from build123d import *

# Parameters (mm, degrees)
SKETCH1_R                       = 7.7978
SKETCH1_R_2                     = 6.57225
SKETCH1_R_3                     = 5.17525
BOSS_EXTRUDE1_DEPTH             = 2.032
BOSS_EXTRUDE2_REACH             = 17.062
BOSS_EXTRUDE2_DIRECTION_2_REACH = 17.062
SKETCH4_W                       = 3.302
SKETCH4_H                       = 2.032
BOSS_EXTRUDE3_DEPTH             = 30.1244
FILLET1_R                       = 2.54
FILLET2_R                       = 2.54
SKETCH5_W                       = 9.0678
SKETCH5_H                       = 2.54
CUT_EXTRUDE1_DEPTH              = 116.84
SKETCH6_R                       = 2.01295
CUT_EXTRUDE2_DEPTH              = 5.7117
SKETCH7_R                       = 1.524
CUT_EXTRUDE3_DEPTH              = 26.9207
CUT_EXTRUDE4_DEPTH              = 116.84
CUT_EXTRUDE4_DEPTH_BACK         = 116.84
SKETCH9_W                       = 42.5577
SKETCH9_H                       = 30.1244
SKETCH9_W_2                     = 39.0017
SKETCH9_H_2                     = 26.5684
BOSS_EXTRUDE4_DEPTH             = 1.778


with BuildPart() as part:
    # Sketch1 → Boss-Extrude1 (new body)
    with BuildSketch(Plane(origin=(0, 0, 0), x_dir=(1, 0, 0), z_dir=(0, 1, 0))):
        with BuildLine():
            ThreePointArc((-23.05685, 9.9822), (-21.568952448, 13.574302448), (-17.97685, 15.0622))
            Line((-17.97685, 15.0622), (17.97685, 15.0622))
            ThreePointArc((17.97685, 15.0622), (21.568952448, 13.574302448), (23.05685, 9.9822))
            Line((23.05685, 9.9822), (23.05685, -9.9822))
            ThreePointArc((23.05685, -9.9822), (21.568952448, -13.574302448), (17.97685, -15.0622))
            Line((17.97685, -15.0622), (-17.97685, -15.0622))
            ThreePointArc((-17.97685, -15.0622), (-21.568952448, -13.574302448), (-23.05685, -9.9822))
            Line((-23.05685, -9.9822), (-23.05685, 9.9822))
        make_face()
        Circle(SKETCH1_R, mode=Mode.SUBTRACT)
        Circle(SKETCH1_R)
        Circle(SKETCH1_R_2, mode=Mode.SUBTRACT)
        Circle(SKETCH1_R_2)
        Circle(SKETCH1_R_3, mode=Mode.SUBTRACT)
    extrude(amount=-BOSS_EXTRUDE1_DEPTH)

    # Sketch2 → Revolve1 (revolve)
    with BuildSketch(Plane(origin=(0, 0, 0), x_dir=(0, 0, -1), z_dir=(1, 0, 0))):
        Polygon((-5.17525, 2.286), (-6.57225, 2.794), (-7.7978, 0), (-5.17525, 0), align=None)
    revolve1 = revolve(axis=Axis((0, 0, 0), (0, 1, 0)))

    # Boss-Extrude2: up to this face of the body (flat: up to its plane)
    boss_extrude2_end = Plane(part.part.faces().sort_by_distance((0, -1.016, 15.0622))[0])
    # Sketch3 → Boss-Extrude2 (add, up to the picked face)
    with BuildSketch(Plane.XY, mode=Mode.PRIVATE) as boss_extrude2_sk1:
        with BuildLine():
            ThreePointArc((-23.05685, -1.27), (-22.684875612, -0.371974388), (-21.78685, 0))
            Line((-21.78685, 0), (-21.27885, 0))
            Line((-21.27885, 0), (-21.27885, -21.717))
            ThreePointArc((-21.27885, -21.717), (-21.650824388, -22.615025612), (-22.54885, -22.987))
            Line((-22.54885, -22.987), (-23.05685, -22.987))
            Line((-23.05685, -22.987), (-32.16275, -22.987))
            Line((-32.16275, -22.987), (-32.16275, -25.9207))
            Line((-32.16275, -25.9207), (-33.94075, -25.9207))
            Line((-33.94075, -25.9207), (-33.94075, -22.479))
            ThreePointArc((-33.94075, -22.479), (-33.568775612, -21.580974388), (-32.67075, -21.209))
            Line((-32.67075, -21.209), (-32.16275, -21.209))
            Line((-32.16275, -21.209), (-23.05685, -21.209))
            Line((-23.05685, -21.209), (-23.05685, -1.27))
        make_face()
    boss_extrude2_tool1 = split(extrude(boss_extrude2_sk1.sketch, amount=BOSS_EXTRUDE2_REACH, mode=Mode.PRIVATE), bisect_by=boss_extrude2_end, keep=Keep.BOTH, mode=Mode.PRIVATE)
    add(boss_extrude2_tool1.solids().sort_by_distance((-32.41675, -21.49748, 0))[0])
    # Sketch3 → Boss-Extrude2 (add, up to the picked face)
    with BuildSketch(Plane.XY, mode=Mode.PRIVATE) as boss_extrude2_sk2:
        with BuildLine():
            Line((21.27885, 0), (21.27885, -21.717))
            ThreePointArc((21.27885, -21.717), (21.650824388, -22.615025612), (22.54885, -22.987))
            Line((22.54885, -22.987), (23.05685, -22.987))
            Line((23.05685, -22.987), (32.16275, -22.987))
            Line((32.16275, -22.987), (32.16275, -25.9207))
            Line((32.16275, -25.9207), (33.94075, -25.9207))
            Line((33.94075, -25.9207), (33.94075, -22.479))
            ThreePointArc((33.94075, -22.479), (33.568775612, -21.580974388), (32.67075, -21.209))
            Line((32.67075, -21.209), (32.16275, -21.209))
            Line((32.16275, -21.209), (23.05685, -21.209))
            Line((23.05685, -21.209), (23.05685, -1.27))
            ThreePointArc((23.05685, -1.27), (22.684875612, -0.371974388), (21.78685, 0))
            Line((21.78685, 0), (21.27885, 0))
        make_face()
    boss_extrude2_tool2 = split(extrude(boss_extrude2_sk2.sketch, amount=BOSS_EXTRUDE2_REACH, mode=Mode.PRIVATE), bisect_by=boss_extrude2_end, keep=Keep.BOTH, mode=Mode.PRIVATE)
    add(boss_extrude2_tool2.solids().sort_by_distance((32.41675, -21.49748, 0))[0])

    # Boss-Extrude2 direction 2: up to this face of the body (flat: up to its plane)
    boss_extrude2_direction_2_end = Plane(part.part.faces().sort_by_distance((0, -1.016, -15.0622))[0])
    # Sketch3 → Boss-Extrude2 direction 2 (add, up to the picked face)
    with BuildSketch(Plane.XY, mode=Mode.PRIVATE) as boss_extrude2_direction_2_sk1:
        with BuildLine():
            ThreePointArc((-23.05685, -1.27), (-22.684875612, -0.371974388), (-21.78685, 0))
            Line((-21.78685, 0), (-21.27885, 0))
            Line((-21.27885, 0), (-21.27885, -21.717))
            ThreePointArc((-21.27885, -21.717), (-21.650824388, -22.615025612), (-22.54885, -22.987))
            Line((-22.54885, -22.987), (-23.05685, -22.987))
            Line((-23.05685, -22.987), (-32.16275, -22.987))
            Line((-32.16275, -22.987), (-32.16275, -25.9207))
            Line((-32.16275, -25.9207), (-33.94075, -25.9207))
            Line((-33.94075, -25.9207), (-33.94075, -22.479))
            ThreePointArc((-33.94075, -22.479), (-33.568775612, -21.580974388), (-32.67075, -21.209))
            Line((-32.67075, -21.209), (-32.16275, -21.209))
            Line((-32.16275, -21.209), (-23.05685, -21.209))
            Line((-23.05685, -21.209), (-23.05685, -1.27))
        make_face()
    boss_extrude2_direction_2_tool1 = split(extrude(boss_extrude2_direction_2_sk1.sketch, amount=-BOSS_EXTRUDE2_DIRECTION_2_REACH, mode=Mode.PRIVATE), bisect_by=boss_extrude2_direction_2_end, keep=Keep.BOTH, mode=Mode.PRIVATE)
    add(boss_extrude2_direction_2_tool1.solids().sort_by_distance((-32.41675, -21.49748, 0))[0])
    # Sketch3 → Boss-Extrude2 direction 2 (add, up to the picked face)
    with BuildSketch(Plane.XY, mode=Mode.PRIVATE) as boss_extrude2_direction_2_sk2:
        with BuildLine():
            Line((21.27885, 0), (21.27885, -21.717))
            ThreePointArc((21.27885, -21.717), (21.650824388, -22.615025612), (22.54885, -22.987))
            Line((22.54885, -22.987), (23.05685, -22.987))
            Line((23.05685, -22.987), (32.16275, -22.987))
            Line((32.16275, -22.987), (32.16275, -25.9207))
            Line((32.16275, -25.9207), (33.94075, -25.9207))
            Line((33.94075, -25.9207), (33.94075, -22.479))
            ThreePointArc((33.94075, -22.479), (33.568775612, -21.580974388), (32.67075, -21.209))
            Line((32.67075, -21.209), (32.16275, -21.209))
            Line((32.16275, -21.209), (23.05685, -21.209))
            Line((23.05685, -21.209), (23.05685, -1.27))
            ThreePointArc((23.05685, -1.27), (22.684875612, -0.371974388), (21.78685, 0))
            Line((21.78685, 0), (21.27885, 0))
        make_face()
    boss_extrude2_direction_2_tool2 = split(extrude(boss_extrude2_direction_2_sk2.sketch, amount=-BOSS_EXTRUDE2_DIRECTION_2_REACH, mode=Mode.PRIVATE), bisect_by=boss_extrude2_direction_2_end, keep=Keep.BOTH, mode=Mode.PRIVATE)
    add(boss_extrude2_direction_2_tool2.solids().sort_by_distance((32.41675, -21.49748, 0))[0])

    # Sketch4 → Boss-Extrude3 (add)
    with BuildSketch(Plane.XY.offset(15.0622)):
        with BuildLine():
            ThreePointArc((-23.05685, -1.27), (-22.684875612, -0.371974388), (-21.78685, 0))
            Line((-21.78685, 0), (-23.05685, 0))
            Line((-23.05685, 0), (-23.05685, -1.27))
        make_face()
        with BuildLine():
            Line((-21.27885, -2.032), (-21.27885, 0))
            Line((-21.27885, 0), (-21.78685, 0))
            ThreePointArc((-21.78685, 0), (-22.684875612, -0.371974388), (-23.05685, -1.27))
            Line((-23.05685, -1.27), (-23.05685, -2.032))
            Line((-23.05685, -2.032), (-21.27885, -2.032))
        make_face()
        with Locations((-19.62785, -1.016)):
            Rectangle(SKETCH4_W, SKETCH4_H)
        Polygon((23.05685, 0), (21.27885, 0), (17.97685, 0), (17.97685, -2.032), (21.27885, -2.032), (23.05685, -2.032), align=None)
    extrude(amount=-BOSS_EXTRUDE3_DEPTH)

    # Fillet1
    fillet1_edges = [part.edges().sort_by_distance(p)[0] for p in [
        (23.05685, 0, 0),
    ]]
    fillet(fillet1_edges, radius=FILLET1_R)

    # Fillet2
    fillet2_edges = [part.edges().sort_by_distance(p)[0] for p in [
        (-23.05685, 0, 0),
    ]]
    fillet(fillet2_edges, radius=FILLET2_R)

    # Sketch5 → Cut-Extrude1 (cut)
    with BuildSketch(Plane.ZY.offset(33.94075)):
        with Locations((0, -24.6507)):
            Rectangle(SKETCH5_W, SKETCH5_H)
    extrude(amount=-CUT_EXTRUDE1_DEPTH, mode=Mode.SUBTRACT)

    # Sketch6 → Cut-Extrude2 (cut, through all)
    with BuildSketch(Plane(origin=(0, -21.209, 0), x_dir=(1, 0, 0), z_dir=(0, 1, 0))):
        with Locations((-28.4734, 0)):
            Circle(SKETCH6_R)
        with Locations((28.4734, 0)):
            Circle(SKETCH6_R)
    extrude(amount=-CUT_EXTRUDE2_DEPTH, mode=Mode.SUBTRACT)

    # Sketch7 → Cut-Extrude3 (cut, through all)
    with BuildSketch(Plane(origin=(0, 0, 0), x_dir=(1, 0, 0), z_dir=(0, 1, 0))):
        with Locations((13.725830849, 0)):
            Circle(SKETCH7_R)
        with Locations((-13.725830849, 0)):
            Circle(SKETCH7_R)
        with Locations((-6.862915424, -11.886918203)):
            Circle(SKETCH7_R)
        with Locations((6.862915424, 11.886918203)):
            Circle(SKETCH7_R)
        with Locations((-6.862915424, 11.886918203)):
            Circle(SKETCH7_R)
        with Locations((6.862915424, -11.886918203)):
            Circle(SKETCH7_R)
    extrude(amount=-CUT_EXTRUDE3_DEPTH, mode=Mode.SUBTRACT)

    # Sketch8 → Cut-Extrude4 (cut, two sides)
    with BuildSketch(Plane.ZY.offset(23.05685)) as cut_extrude4_sk:
        Polygon((-15.0622, -2.54), (-9.0678, -25.9207), (-15.0622, -25.9207), align=None)
        Polygon((9.0678, -25.9207), (15.0622, -2.54), (15.0622, -25.9207), align=None)
    extrude(amount=CUT_EXTRUDE4_DEPTH, mode=Mode.SUBTRACT)
    extrude(cut_extrude4_sk.sketch, amount=-CUT_EXTRUDE4_DEPTH_BACK, mode=Mode.SUBTRACT)

    # Mirror4: Revolve1 across plane
    add(revolve1.mirror(Plane.ZX.offset(-1.016)))

    # Sketch9 → Boss-Extrude4 (add)
    with BuildSketch(Plane.XZ.offset(2.032)):
        Rectangle(SKETCH9_W, SKETCH9_H)
        Rectangle(SKETCH9_W_2, SKETCH9_H_2, mode=Mode.SUBTRACT)
    extrude(amount=BOSS_EXTRUDE4_DEPTH)


solid = part.part
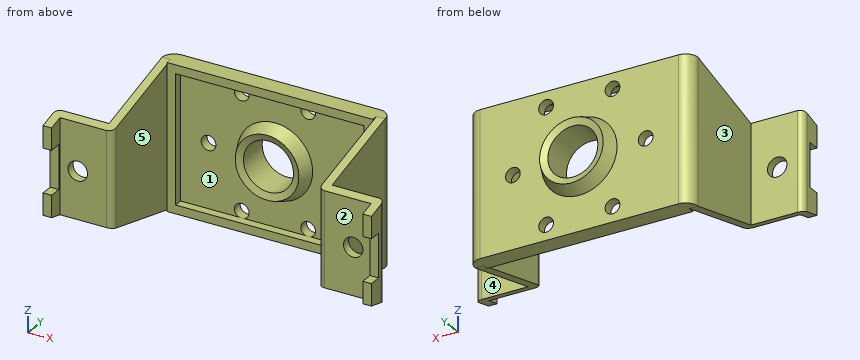
Work out the finished part from the listing and answer in its coordinate system (mm). Face numbers are marked on the shaded views. A direction names the side the tool comes from. Round coordinates to 2 decimals unless told otherwise and drop trailing zeros. Loops run counter-clockwise (first coordinate to the right, second up) from the corner with the lowest first, then second, coordinate; pieces in that order, holes last. Notation, with made-up numbers: (55, 67) - (73, 67) arc R18 ccw to (73, 97) - close; hole circle Ø5 at (40, 30.25). An arc over 180 degrees is marked (long way). Use one line per item in the form item = value. Start each with the question number.
(1) Find section A-A on x = 0. Determine the outline of the cut face in (y, z).
(2) Which of the six approach directions +Z, -Z, +X, -X, +Y, -Y give full straight-line access (tool end or side, diameter ignored) to the marked faces 3, 4 and 5?
(3) Find section C-C on y = -10. Determine the outline of the cut face in (x, z).
(4) Determine the mould class of the marked faces 1 and 2 for opening direction Z: +Z half, -Z half, draft (parallel to the pull), parting line (faces both ways), or undercut.
(5) Consider line 1 (X direction, y = -4, z = -7.5); line 2 (X direction, y = -22.55, z = 0); line 3 (X direction, y = -0.5, z = 12). Determine where each line is inside the solid, lowest interval first.
(6) Find section D-D on x = 11.5. Determine the outline of the cut face in (y, z), and give its area (3 significant figures).
(7) Flat-ended cylindrical pins translate along their axes: P1, Ø5, axis at y = -2, z = -4, coming from the +X side; P2, Ø6, axis at x = 0, z = 2.5, coming from the +Y side; P3, Ø0.5, axis at x = -33, y = -24.5, coming from the -Z side. Find the tip coordinate at first contact, or state that the pin passes through.
(8) Find section B-B on z = 11. Determine the outline of the cut face in (x, y), and give its area (3 significant figures).
Answer list:
q1.outline = (-4.83, -6.57) - (-2.03, -7.8) - (-2.03, -13.28) - (-3.81, -13.28) - (-3.81, -15.06) - (0, -15.06) - (0, -7.8) - (2.79, -6.57) - (2.29, -5.18) - (-4.32, -5.18) - close; (-4.83, 6.57) - (-4.32, 5.18) - (2.29, 5.18) - (2.79, 6.57) - (0, 7.8) - (0, 15.06) - (-3.81, 15.06) - (-3.81, 13.28) - (-2.03, 13.28) - (-2.03, 7.8) - close
q2.face_3 = +Z, -Z, -X, +Y
q2.face_4 = +Z, -Z, +X, +Y
q2.face_5 = +Z, -Z, -Y
q3.outline = (-23.06, -13.15) - (-21.28, -13.15) - (-21.28, 13.15) - (-23.06, 13.15) - close; (21.28, -13.15) - (23.06, -13.15) - (23.06, 13.15) - (21.28, 13.15) - close
q4.face_1 = undercut
q4.face_2 = draft
q5.line_1 = -23.06 to -21.28, 21.28 to 23.06
q5.line_2 = -33.94 to -30.49, -26.46 to -21.59, 21.59 to 26.46, 30.49 to 33.94
q5.line_3 = -22.03 to -8.38, -5.34 to 5.34, 8.38 to 22.03
q6.outline = (-3.81, -15.06) - (0, -15.06) - (0, 15.06) - (-3.81, 15.06) - (-3.81, 13.28) - (-2.03, 13.28) - (-2.03, -13.28) - (-3.81, -13.28) - close
q6.area = 67.5 mm^2
q7.P1 = 23.06
q7.P2 = 2.4
q7.P3 = -9.5
q8.outline = (-23.06, -18.38) - (-21.28, -18.38) - (-21.28, -3.81) - (-19.5, -3.81) - (-19.5, -2.03) - (-8.1, -2.03) - (-8.1, 0) - (-20.52, 0) arc R2.54 ccw to (-23.06, -2.54) - close; (-5.62, -2.03) - (5.62, -2.03) - (5.62, 0) - (-5.62, 0) - close; (8.1, -2.03) - (19.5, -2.03) - (19.5, -3.81) - (21.28, -3.81) - (21.28, -18.38) - (23.06, -18.38) - (23.06, -2.54) arc R2.54 ccw to (20.52, 0) - (8.1, 0) - close
q8.area = 145 mm^2
